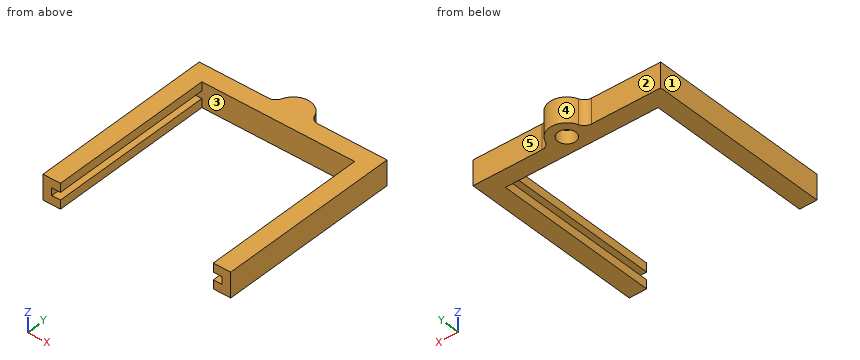
Solid Edge part; units mm, degrees
sketch "Sketch1" plane through (0, 0, 0) normal (0, -1, 0) x (1, 0, 0)
  line L0 (17.5, 2) -> (17.5, 0)
  line L1 (17.5, 0) -> (21.5, 0)
  line L2 (21.5, 0) -> (21.5, 5.7)
  line L3 (21.5, 5.7) -> (17.5, 5.7)
  line L4 (17.5, 5.7) -> (17.5, 3.7)
  line L5 (17.5, 3.7) -> (19.5, 3.7)
  line L6 (19.5, 3.7) -> (19.5, 2)
  line L7 (19.5, 2) -> (17.5, 2)
  line L8 (-21.5, 0) -> (-21.5, 5.7)
  line L9 (-21.5, 5.7) -> (-17.5, 5.7)
  line L10 (-17.5, 5.7) -> (-17.5, 3.7)
  line L11 (-17.5, 3.7) -> (-19.5, 3.7)
  line L12 (-19.5, 3.7) -> (-19.5, 2)
  line L13 (-19.5, 2) -> (-17.5, 2)
  line L14 (-17.5, 2) -> (-17.5, 0)
  line L15 (-17.5, 0) -> (-21.5, 0)
extrude "Protrusion1" add sketch "Sketch1" against normal blind 38
sketch "Sketch2" plane through (-19.2, 19, 5.7) normal (0, 0, 1) x (0, 1, 0)
  line L0 (23, 2.3) -> (23, -40.7)
  line L1 (23, -40.7) -> (19, -40.7)
  line L2 (19, -40.7) -> (19, 2.3)
  line L3 (19, 2.3) -> (23, 2.3)
extrude "Protrusion2" add sketch "Sketch2" against normal up to surface (5.7 mm away)
sketch "Sketch3" plane through (0, 21, 0) normal (0, 0, -1) x (0, 1, 0)
  arc A0 (21, 4) -> (21, -4) centre (21, 0) cw
  line L0 (21, -4) -> (21, 4)
extrude "Protrusion3" add sketch "Sketch3" against normal up to surface (5.7 mm away)
hole "Agujero_1" at (0, 42, 0) direction (0, 0, 1) diameter 4.1 depth 3
fillet "Redondeo_1" radius 2 2 edges at (-4, 42, 2.85) (4, 42, 2.85)
Design review of the part built by this model. Coordinates are the model's own, in mm. Face numbers are marked on the shaded views. A direction names the side the tool comes from. Round coordinates to 2 decimals unless told otherwise and drop trailing zeros. Write each loop counter-clockwise with the first axis right and the second up, starting at its lowest first coordinate (ties: lowest second). Pieces come first, ordered by that corner, then holes. Notation, with made-up numbers: (45, 83.25) -> (100, 83.25) arc R25 ccw to (100, 106.25) -> close; hole circle Ø3 at (40.25, 85). An arc over 180 degrees is marked (long way). One line per item, written item: value. Start each with the question number.
Q1. To check wall thickness, follow probe 1 along Y at (x, z) = (0, 1.9); probe 2 along X at (y, z) = (35, 2.85); probe 3 along X at (y, z) = (10, 4.45). State the ranges of each line that lie inside material, in increasing order.
Q2. Add section A-A (z = 4.45). Give the boundary of the cut face in (x, y), then the cut area to 3 significant figures.
Q3. Tool access review of the marked faces 1 and 2: name each direction out of +Z, -Z, +X, -X, +Y, -Y from which nothing blocks a thin tool from reaching the whole face with its end or side.
Q4. Insertion check: P1, Ø1.7, axis at x = -9, z = 3.5, coming from the -Y side; P2, Ø3.5, axis at x = 0, y = 42, coming from the -Z side; P3, Ø3, axis at x = 12.5, z = 3, coming from the +Y side. Each pin has a flat end and moves straight along its axis. Give the tip position at first contact, or say it passes through.
Q5. Add section D-D (x = 0). Give the boundary of the cut face in (y, z).
Q6. Add section B-B (y = 13.5). Give the boundary of the cut face in (x, z), then the cut area to 3 significant figures.
Q7. Add section C-C (z = 1.1). Give the boundary of the cut face in (x, y), then the cut area to 3 significant figures.
Q8. The part is to be moulded in two halves that separate along X. For the marked faces 3, 4 and 5, say which applies: pulls with the +X half, pulls with the -X half, needs draft (parallel to the pull), parting line crosses it, or undercut.
Response:
1. probe 1: y = 38 to 39.95, 44.05 to 46
1. probe 2: x = -21.5 to -19.5, 19.5 to 21.5
1. probe 3: x = -21.5 to -17.5, 17.5 to 21.5
2. outline: (-21.5, 0) -> (-17.5, 0) -> (-17.5, 38) -> (17.5, 38) -> (17.5, 0) -> (21.5, 0) -> (21.5, 42) -> (5.66, 42) arc R2 cw to (3.77, 43.33) arc R4 ccw to (-3.77, 43.33) arc R2 cw to (-5.66, 42) -> (-21.5, 42) -> close
2. area: 502 mm^2
3. face 1: +Z, -Z, -X, +Y, -Y
3. face 2: +Z, -Z, -X, +Y
4. P1: stops at y = 38
4. P2: stops at z = 3
4. P3: stops at y = 42
5. outline: (38, 0) -> (39.95, 0) -> (39.95, 3) -> (44.05, 3) -> (44.05, 0) -> (46, 0) -> (46, 5.7) -> (38, 5.7) -> close
6. outline: (-21.5, 0) -> (-17.5, 0) -> (-17.5, 2) -> (-19.5, 2) -> (-19.5, 3.7) -> (-17.5, 3.7) -> (-17.5, 5.7) -> (-21.5, 5.7) -> close; (17.5, 0) -> (21.5, 0) -> (21.5, 5.7) -> (17.5, 5.7) -> (17.5, 3.7) -> (19.5, 3.7) -> (19.5, 2) -> (17.5, 2) -> close
6. area: 38.8 mm^2
7. outline: (-21.5, 0) -> (-17.5, 0) -> (-17.5, 38) -> (17.5, 38) -> (17.5, 0) -> (21.5, 0) -> (21.5, 42) -> (5.66, 42) arc R2 cw to (3.77, 43.33) arc R4 ccw to (-3.77, 43.33) arc R2 cw to (-5.66, 42) -> (-21.5, 42) -> close; hole circle Ø4.1 at (0, 42)
7. area: 489 mm^2
8. face 3: undercut
8. face 4: parting line crosses it
8. face 5: needs draft
